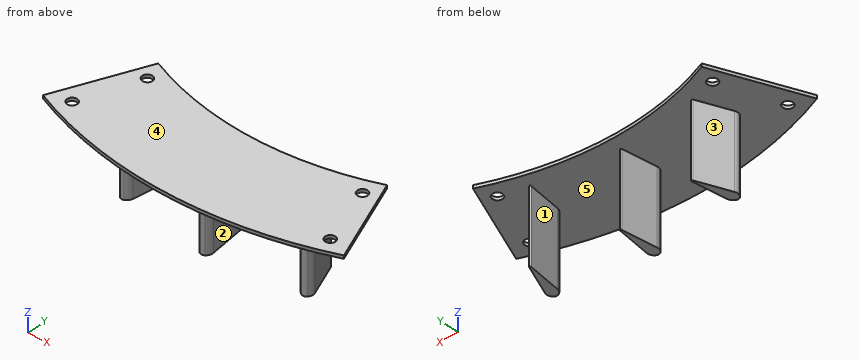
from build123d import *

# Parameters (mm, degrees)
BOSS_EXTRUDE1_START      = -5
BOSS_EXTRUDE1_DEPTH      = 1
BOSS_EXTRUDE2_START      = -5
BOSS_EXTRUDE2_DEPTH      = 5
BOSS_EXTRUDE3_DEPTH      = 1
BOSS_EXTRUDE3_DEPTH_BACK = 6
BOSS_EXTRUDE4_DEPTH      = 23.5
CUT_EXTRUDE1_START       = -6
CUT_EXTRUDE1_DEPTH       = 6
CUT_EXTRUDE2_DEPTH       = 137.064243179
CUT_EXTRUDE2_DEPTH_BACK  = 137.064243179
SKETCH5_R                = 1.6


with BuildPart() as part:
    # Sketch1 → Boss-Extrude1 (new body)
    with BuildSketch(Plane.XY.offset(BOSS_EXTRUDE1_START)):
        with BuildLine():
            Line((-47.835429046, -115.484941564), (-36.354926075, -87.768555589))
            ThreePointArc((-36.354926075, -87.768555589), (0, -95), (36.354926075, -87.768555589))
            Line((36.354926075, -87.768555589), (47.835429046, -115.484941564))
            ThreePointArc((47.835429046, -115.484941564), (0, -125), (-47.835429046, -115.484941564))
        make_face()
        with BuildLine():
            Line((-26.038476963, -106.101650399), (-23.955923749, -97.86049365))
            ThreePointArc((-23.955923749, -97.86049365), (0, -100.75), (23.955923749, -97.86049365))
            Line((23.955923749, -97.86049365), (26.038476963, -106.101650399))
            ThreePointArc((26.038476963, -106.101650399), (0, -109.25), (-26.038476963, -106.101650399))
        make_face(mode=Mode.SUBTRACT)
    extrude(amount=-BOSS_EXTRUDE1_DEPTH)



with BuildPart() as body_2:
    # Sketch1<3> → Boss-Extrude2 (new body)
    with BuildSketch(Plane.XY.offset(BOSS_EXTRUDE2_START)):
        with BuildLine():
            ThreePointArc((-23.955923749, -97.86049365), (0, -100.75), (23.955923749, -97.86049365))
            Line((23.955923749, -97.86049365), (26.038476963, -106.101650399))
            ThreePointArc((26.038476963, -106.101650399), (0, -109.25), (-26.038476963, -106.101650399))
            Line((-26.038476963, -106.101650399), (-23.955923749, -97.86049365))
        make_face()
    extrude(amount=BOSS_EXTRUDE2_DEPTH)


with BuildPart() as part_1:
    add(part.part)

    add(body_2.part)  # Boss-Extrude3 merges body 2
    # Sketch1<4> → Boss-Extrude3 (add, two sides: drawn at the far end of the back side and taken through both)
    with BuildSketch(Plane.XY.offset(-BOSS_EXTRUDE3_DEPTH_BACK)):
        with BuildLine():
            ThreePointArc((-23.955923749, -97.86049365), (0, -100.75), (23.955923749, -97.86049365))
            Line((23.955923749, -97.86049365), (26.038476963, -106.101650399))
            ThreePointArc((26.038476963, -106.101650399), (0, -109.25), (-26.038476963, -106.101650399))
            Line((-26.038476963, -106.101650399), (-23.955923749, -97.86049365))
        make_face()
    extrude(amount=BOSS_EXTRUDE3_DEPTH + BOSS_EXTRUDE3_DEPTH_BACK)

    # Sketch3 → Boss-Extrude4 (add)
    with BuildSketch(Plane(origin=(0, 0, -6), x_dir=(-1, 0, 0), z_dir=(0, 0, -1))):
        with BuildLine():
            Line((-25.529686705, -96.235678696), (-26.946588628, -106.998117309))
            ThreePointArc((-26.946588628, -106.998117309), (-27.363549694, -108.035848526), (-28.228626172, -108.744639958))
            ThreePointArc((-28.228626172, -108.744639958), (-29.159731718, -108.825600307), (-29.9256126, -108.289933815))
            ThreePointArc((-29.9256126, -108.289933815), (-30.32039509, -107.24356419), (-30.162628357, -106.136382061))
            Line((-30.162628357, -106.136382061), (-26.008482111, -96.107385854))
            ThreePointArc((-26.008482111, -96.107385854), (-25.695897738, -95.898395904), (-25.529686705, -96.235678696))
        make_face()
        with BuildLine():
            Line((0.24784274, -99.564096598), (1.664744663, -110.326535211))
            ThreePointArc((1.664744663, -110.326535211), (1.530575804, -111.436824058), (0.878424814, -112.345362277))
            ThreePointArc((0.878424814, -112.345362277), (0, -112.664551817), (-0.878424814, -112.345362277))
            ThreePointArc((-0.878424814, -112.345362277), (-1.530575804, -111.436824058), (-1.664744663, -110.326535211))
            Line((-1.664744663, -110.326535211), (-0.24784274, -99.564096598))
            ThreePointArc((-0.24784274, -99.564096598), (0, -99.281325019), (0.24784274, -99.564096598))
        make_face()
        with BuildLine():
            Line((26.008482111, -96.107385854), (30.162628357, -106.136382061))
            ThreePointArc((30.162628357, -106.136382061), (30.32039509, -107.24356419), (29.9256126, -108.289933815))
            ThreePointArc((29.9256126, -108.289933815), (29.159731718, -108.825600307), (28.228626172, -108.744639958))
            ThreePointArc((28.228626172, -108.744639958), (27.363549694, -108.035848526), (26.946588628, -106.998117309))
            Line((26.946588628, -106.998117309), (25.529686705, -96.235678696))
            ThreePointArc((25.529686705, -96.235678696), (25.695897738, -95.898395904), (26.008482111, -96.107385854))
        make_face()
    extrude(amount=BOSS_EXTRUDE4_DEPTH)

    # Sketch4 → Cut-Extrude1 (cut)
    with BuildSketch(Plane.XY.offset(1).offset(CUT_EXTRUDE1_START)):
        with BuildLine():
            Line((-23.955923749, -97.86049365), (-26.038476963, -106.101650399))
            ThreePointArc((-26.038476963, -106.101650399), (0, -109.25), (26.038476963, -106.101650399))
            Line((26.038476963, -106.101650399), (23.955923749, -97.86049365))
            ThreePointArc((23.955923749, -97.86049365), (0, -100.75), (-23.955923749, -97.86049365))
        make_face()
    extrude(amount=CUT_EXTRUDE1_DEPTH, mode=Mode.SUBTRACT)

    # Sketch5 → Cut-Extrude2 (cut, two sides: drawn at the far end of the back side and taken through both)
    with BuildSketch(Plane.XY.offset(-5).offset(-CUT_EXTRUDE2_DEPTH_BACK)):
        with Locations((-34.202014333, -93.969262079)):
            Circle(SKETCH5_R)
        with Locations((-41.042417199, -112.763114494)):
            Circle(SKETCH5_R)
        with Locations((41.042417199, -112.763114494)):
            Circle(SKETCH5_R)
        with Locations((34.202014333, -93.969262079)):
            Circle(SKETCH5_R)
    extrude(amount=CUT_EXTRUDE2_DEPTH + CUT_EXTRUDE2_DEPTH_BACK, mode=Mode.SUBTRACT)


solid = part_1.part
Design review of the part built by this model. Coordinates are the model's own, in mm. Face numbers are marked on the shaded views. A direction names the side the tool comes from. Round coordinates to 2 decimals unless told otherwise and drop trailing zeros. Order: outer loops, then holes, each group sorted by start corner. A loop starts at its lowest first (then second) coordinate and runs counter-clockwise, first axis right, second up.
1) For L1, parallel to X at y = -106, z = -23; L2, parallel to X at y = -100, z = -17; L3, parallel to Z at x = -29, y = -96, list the stretches that pass through material, from the lowest coordinate up.
The answers:
L1: x = -30.11 to -26.82, -1.1 to 1.1, 26.82 to 30.11
L2: x = -27.62 to -26.03, -0.31 to 0.31, 26.03 to 27.62
L3: z = -6 to -5
2) Machinability: for the marked faces 1 and 2, which of the approach directions +Z, -Z, +X, -X, +Y, -Y give a long, thin tool a straight path to every point of the face, cutting with its end or side? Answer none if there is none.
The answers:
face 1: -Z, -Y
face 2: -Z, +Y
3) Consider section B-B (x = -9.5). State the section outline as (y, z) points, plus the area to 3 significant figures.
The answers:
outline: (-124.64, -6) - (-94.52, -6) - (-94.52, -5) - (-124.64, -5) - close
area: 30.1 mm2
4) Clearance check with flat-ended pins moving along their axes: pin 1 Ø4 at (y, z) = (-99.5, -12) entering from -X; pin 2 Ø1.9 at (x, y) = (-41.04, -112.76) entering from +Z; pin 3 Ø1.5 at (x, y) = (-17, -115) entering from -Z; pin 4 Ø12 at (y, z) = (-114.5, -18) entering from +X. State where each tip first meets the part, or that it passes through.
The answers:
pin 1: stops at x = -28.24
pin 2: passes through
pin 3: stops at z = -6
pin 4: stops at x = 29.74
5) Draft analysis for pull direction X (two halves, no side actions). For the marked faces 3, 4 and 5, state which applies: released by +X, released by -X, zero draft, split by the parting line, or undercut.
The answers:
face 3: released by -X
face 4: zero draft
face 5: undercut
6) Consider section A-A (z = -17.75). State the section outline as (x, y) points.
The answers:
outline: (-30.16, -106.14) arc R2.25 ccw to (-29.93, -108.29) arc R1.37 ccw to (-28.23, -108.74) arc R2.25 ccw to (-26.95, -107) - (-25.53, -96.24) arc R0.25 ccw (long way) to (-26.01, -96.11) - close; (-1.66, -110.33) arc R2.25 ccw to (-0.88, -112.35) arc R1.37 ccw to (0.88, -112.35) arc R2.25 ccw to (1.66, -110.33) - (0.25, -99.56) arc R0.25 ccw (long way) to (-0.25, -99.56) - close; (25.53, -96.24) - (26.95, -107) arc R2.25 ccw to (28.23, -108.74) arc R1.37 ccw to (29.93, -108.29) arc R2.25 ccw to (30.16, -106.14) - (26.01, -96.11) arc R0.25 ccw (long way) to start
